Geometry: final body of the model. Coordinates: model frame, mm. A direction names the side the tool comes from. Round coordinates to 2 decimals unless told otherwise and drop trailing zeros. Loops run counter-clockwise (first coordinate to the right, second up) from the corner with the lowest first, then second, coordinate; pieces in that order, holes last. Notation, with made-up numbers: (-33.75, -6.5) -> (14.25, -6.5) arc R5 ccw to (14.25, 0.5) -> close; hole circle Ø5 at (42, 13.25). An arc over 180 degrees is marked (long way). Answer in a Markdown table with one row per item.
```python
from build123d import *

# Parameters (mm, degrees)
F1_DEPTH = 25
F0_W     = 10
F0_H     = 7.5
F2_DEPTH = 10
F3_DEPTH = 3.125
F5_R     = 2.5


with BuildPart() as f1:
    # F0 (on Front) → F1 (new body, symmetric)
    with BuildSketch(Plane.XZ):
        Polygon((-16.25, -3.75), (16.25, -3.75), (16.25, 3.75), (8.75, 3.75), (-16.25, 3.75), align=None)
    extrude(amount=F1_DEPTH, both=True)

    # F0 (on Front) → F2 (join, symmetric)
    with BuildSketch(Plane.XZ):
        with Locations((28.75, 20.63)):
            Rectangle(F0_W, F0_H)
        with BuildLine():
            Line((8.75, 3.75), (16.25, 3.75))
            Line((16.25, 3.75), (16.25, 10.63))
            ThreePointArc((16.25, 10.63), (18.080583, 15.049417), (22.5, 16.88))
            Line((22.5, 16.88), (23.75, 16.88))
            Line((23.75, 16.88), (23.75, 24.38))
            Line((23.75, 24.38), (22.5, 24.38))
            add(Edge.make_bspline(
                [(20.527115, 24.237727), (21.188051, 24.296236), (21.846037, 24.343663), (22.5, 24.38)],
                knots=[42.021678, 42.021678, 42.021678, 42.021678, 43.899424, 43.899424, 43.899424, 43.899424], degree=3))
            ThreePointArc((20.527115, 24.237727), (12.103133, 19.628204), (8.75, 10.63))
            Line((8.75, 10.63), (8.75, 3.75))
        make_face()
    extrude(amount=F2_DEPTH, both=True)

    # F0 (on Front) → F3 (join, symmetric)
    with BuildSketch(Plane.XZ):
        with BuildLine():
            add(Edge.make_bspline(
                [(-16.25, 3.75), (-10.531949, 16.068907), (5.736173, 22.928358), (20.527115, 24.237727)],
                knots=[0, 0, 0, 0, 42.021678, 42.021678, 42.021678, 42.021678], degree=3))
            Line((-16.25, 3.75), (8.75, 3.75))
            Line((8.75, 3.75), (8.75, 10.63))
            ThreePointArc((8.75, 10.63), (12.103133, 19.628204), (20.527115, 24.237727))
        make_face()
    extrude(amount=F3_DEPTH, both=True)

    # F0 (on Front) → F4 (revolve)
    with BuildSketch(Plane.XZ):
        Polygon((33.75, 24.38), (33.75, 16.88), (33.75, 15), (43.75, 15), (43.75, 26.25), (33.75, 26.25), align=None)
    revolve(axis=Axis((33.75, 0, 20.625), (0, 0, 1)))

    # F5
    f5_edges = [f1.edges().sort_by_distance(p)[0] for p in [
        (16.25, -25, 0),
        (-16.25, -25, 0),
        (16.25, 25, 0),
        (-16.25, 25, 0),
    ]]
    fillet(f5_edges, radius=F5_R)


solid = f1.part
```
Item 1: Ray query, L1, parallel to Z at x = -7, y = -7; L2, parallel to Z at x = 24, y = 8.5; L3, parallel to Y at x = 5, z = 17.5 (3 decimals). Return the intervals inside material, ascending.
Ans:
| item | result |
|---|---|
| L1 | -3.75 to 3.75 |
| L2 | 16.88 to 24.38 |
| L3 | -3.125 to 3.125 |
Item 2: First-contact query: P1, Ø3.5, axis at y = 5.5, z = 7.5, coming from the -X side; P2, Ø5.5, axis at x = 29, y = -4, coming from the -Z side; P3, Ø10.5, axis at x = 18, z = 10, coming from the +Y side; P4, Ø3, axis at x = -2, z = 21, coming from the -Y side. Flat tips, straight axial feed; report the tip coordinate or a pass-through.
Ans:
| item | result |
|---|---|
| P1 | x = 8.75 |
| P2 | z = 15 |
| P3 | y = 10 |
| P4 | through |
Item 3: Section query A-A, the plane x = 27.5. Output: boundary loops of the cut face in (y, z), and give its area (3 significant figures).
Ans:
| item | result |
|---|---|
| outline | (-10, 16.88) -> (-7.81, 16.88) -> (-7.81, 15) -> (7.81, 15) -> (7.81, 16.88) -> (10, 16.88) -> (10, 24.38) -> (7.81, 24.38) -> (7.81, 26.25) -> (-7.81, 26.25) -> (-7.81, 24.38) -> (-10, 24.38) -> close |
| area | 209 mm2 |
Item 4: Set-up query: faces 1 (the flat face through (34, 0, 15)), 2 (the flat face through (23.6, -0.8, 24.38)), 3 (the flat face through (-2, 3.125, 12)). Return all of +Z, -Z, +X, -X, +Y, -Y with unobstructed straight access to the full face (end or side cutting, diameter ignored); none if empty.
Ans:
| item | result |
|---|---|
| face 1 | -Z, +X, +Y, -Y |
| face 2 | +Z, -X |
| face 3 | +Z, -X, +Y |
Item 5: Section query B-B, the plane y = 13.5. Output: boundary loops of the cut face in (x, z).
Ans:
| item | result |
|---|---|
| outline | (-16.25, -3.75) -> (16.25, -3.75) -> (16.25, 3.75) -> (-16.25, 3.75) -> close |
Item 6: Section query C-C, the plane x = 37. Output: boundary loops of the cut face in (y, z).
Ans:
| item | result |
|---|---|
| outline | (-9.46, 15) -> (9.46, 15) -> (9.46, 26.25) -> (-9.46, 26.25) -> close |
Item 7: Mould query, pull axis X, two halves, no side actions, for faces 4 (the cylindrical face through (18.03, -0.14, 15)), 5 (the flat face through (0, 25, 0)), 6 (the cylindrical face through (-15.537, 24.248, -0.053)). Classes: released by +X, released by -X, zero draft, split by the parting line, or undercut.
Ans:
| item | result |
|---|---|
| face 4 | undercut |
| face 5 | zero draft |
| face 6 | released by -X |
